Here's how the part is built. I have some questions about the finished solid (model axes, mm). Face numbers are marked on the shaded views. A direction names the side the tool comes from. Give positions to 0.01 mm unless a question says otherwise; leave off trailing zeros. Loops run counter-clockwise (first coordinate to the right, second up) from the corner with the lowest first, then second, coordinate; pieces in that order, holes last. Notation, with made-up numbers: (41.5, 85.25) - (84.5, 85.25) arc R24 cw to (84.5, 105.25) - close; hole circle Ø2 at (12, 60). An arc over 180 degrees is marked (long way). Use one line per item in the form item = value.
from build123d import *

# Parameters (mm, degrees)
SKETCH1_W                     = 63.5
SKETCH1_H                     = 63.5
BOSS_EXTRUDE1_DEPTH           = 50.8
SKETCH2_R                     = 2.54
BOSS_EXTRUDE2_DEPTH           = 12.7
SKETCH3_R                     = 12.7
BOSS_EXTRUDE3_DEPTH           = 15.24
BOSS_EXTRUDE3_TAPER           = 9
BOSS_EXTRUDE3_OTHER_WAY_DEPTH = 10.16
BOSS_EXTRUDE3_OTHER_WAY_TAPER = -9
BOSS_EXTRUDE4_START           = -25.4
SKETCH4_R                     = 18.536300075
BOSS_EXTRUDE4_DEPTH           = 3.175
BOSS_EXTRUDE4_TAPER           = 58
CHAMFER1_SIZE                 = 1.27
CHAMFER1_SIZE_2               = 1.527812426
SKETCH6_W                     = 38.1
SKETCH6_H                     = 10.16
BOSS_EXTRUDE6_DEPTH           = 6.35
BOSS_EXTRUDE7_DEPTH           = 6.35
BOSS_EXTRUDE7_DEPTH_BACK      = 6.35
SKETCH7_W                     = 1.5875
SKETCH7_H                     = 12.7
FILLET1_R                     = 1.27
SKETCH8_R                     = 4.445
CUT_EXTRUDE1_DEPTH            = 7.62


with BuildPart() as part:
    # Sketch1 → Boss-Extrude1 (new body)
    with BuildSketch(Plane.XY):
        Rectangle(SKETCH1_W, SKETCH1_H)
    extrude(amount=BOSS_EXTRUDE1_DEPTH)

    # Sketch2 → Boss-Extrude2 (add)
    with BuildSketch(Plane(origin=(0, 0, 0), x_dir=(-1, 0, 0), z_dir=(0, 0, -1))):
        with Locations(Location((0, 0, 0), (0, 0, 180))):
            Circle(SKETCH2_R)
    extrude(amount=BOSS_EXTRUDE2_DEPTH)

    # Sketch3 → Boss-Extrude3 (add)
    with BuildSketch(Plane(origin=(0, 0, -12.7), x_dir=(-1, 0, 0), z_dir=(0, 0, -1))):
        Circle(SKETCH3_R)
    extrude(amount=BOSS_EXTRUDE3_DEPTH, taper=BOSS_EXTRUDE3_TAPER)

    # Sketch3 → Boss-Extrude3 other way (add)
    with BuildSketch(Plane(origin=(0, 0, -12.7), x_dir=(-1, 0, 0), z_dir=(0, 0, -1))):
        Circle(SKETCH3_R)
    extrude(amount=-BOSS_EXTRUDE3_OTHER_WAY_DEPTH, taper=BOSS_EXTRUDE3_OTHER_WAY_TAPER)

    # Sketch4 → Boss-Extrude4 (add)
    with BuildSketch(Plane(origin=(0, 0, -27.94), x_dir=(-1, 0, 0), z_dir=(0, 0, -1)).offset(BOSS_EXTRUDE4_START)):
        Circle(SKETCH4_R)
    extrude(amount=BOSS_EXTRUDE4_DEPTH, taper=BOSS_EXTRUDE4_TAPER)

    # Chamfer1
    # the kernel refuses this chamfer: 1.527812426, 1.27 mm, written as the material it takes off along each edge
    with BuildSketch(Plane(origin=(0, 0, -27.94), x_dir=(-1, 0, 0), z_dir=(0, 1, 0))) as chamfer1_piece_1:
        Polygon((10.286221129 + CHAMFER1_SIZE * 0.15643446504, CHAMFER1_SIZE * 0.987688340595), (10.286221129 - CHAMFER1_SIZE_2, 0), (10.286221129, 0), align=None)
    revolve(axis=Axis((0, 0, -27.94), (0, 0, 1)), mode=Mode.SUBTRACT)

    # Sketch6 → Boss-Extrude6 (add)
    with BuildSketch(Plane.XY.offset(50.8)):
        with Locations((0, 14.933737581)):
            Rectangle(SKETCH6_W, SKETCH6_H)
    extrude(amount=BOSS_EXTRUDE6_DEPTH)

    # Sketch7 → Boss-Extrude7 (add, two sides: drawn at the far end of the back side and taken through both)
    with BuildSketch(Plane.XY.offset(57.15).offset(-BOSS_EXTRUDE7_DEPTH_BACK)):
        with Locations((-9.557292348, 14.933737581)):
            Rectangle(SKETCH7_W, SKETCH7_H)
        with Locations((-0.131236763, 14.933737581)):
            Rectangle(SKETCH7_W, SKETCH7_H)
        with Locations((10.440040529, 14.933737581)):
            Rectangle(SKETCH7_W, SKETCH7_H)
    extrude(amount=BOSS_EXTRUDE7_DEPTH + BOSS_EXTRUDE7_DEPTH_BACK)

    # Fillet1
    fillet1_edges = [part.edges().sort_by_distance(p)[0] for p in [
        (10.440040529, 21.283737581, 63.5),
        (10.440040529, 8.583737581, 63.5),
        (-0.131236763, 21.283737581, 63.5),
        (-0.131236763, 8.583737581, 63.5),
        (-9.557292348, 21.283737581, 63.5),
        (-9.557292348, 8.583737581, 63.5),
    ]]
    fillet(fillet1_edges, radius=FILLET1_R)

    # Sketch8 → Cut-Extrude1 (cut)
    with BuildSketch(Plane(origin=(0, 31.75, 0), x_dir=(1, 0, 0), z_dir=(0, 1, 0))):
        with Locations(Location((9.570348057, -25.239963614, 0), (0, 0, 270))):
            Circle(SKETCH8_R)
    extrude(amount=-CUT_EXTRUDE1_DEPTH, mode=Mode.SUBTRACT)


solid = part.part
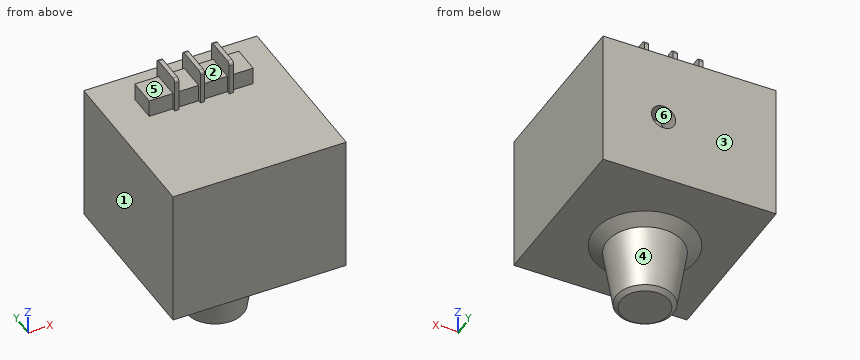
(1) If we section it at D-D (z = -15): List the corners of the cut face in (x, y) for me, plus the area to 3 significant figures.
Geometry says:
outline = circle Ø24.67 at (0, 0)
area = 478 mm²
(2) For P1, Ø0.8, axis at x = 10.5, z = 55.5, coming from the -Y side; P2, Ø12, axis at x = -9.5, y = -22.5, coming from the -Z side; P3, Ø0.8, axis at x = -9.5, z = 55, coming from the +Y side, each with a flat end and sliding along its axis, tell me the tip position at first contact or that it passes through.
Geometry says:
P1 = 8.58
P2 = -2.61
P3 = 21.28
(3) Thinking about a two-plate mould opening in X: for the marked faces 1, 2 and 3, which applies, pulls with the +X half, pulls with the -X half, needs draft (parallel to the pull), parting line crosses it, or undercut?
Geometry says:
face_1 = pulls with the -X half
face_2 = undercut
face_3 = needs draft
(4) If we section it at B-B (x = -23.5): List the corners of the cut face in (y, z) for me.
Geometry says:
outline = (-31.75, 0) - (31.75, 0) - (31.75, 50.8) - (-31.75, 50.8) - close
(5) If we section it at A-A (y = 26): List the corners of the cut face in (x, z) for me (3 decimals).
Geometry says:
outline = (-31.75, 0) - (31.75, 0) - (31.75, 50.8) - (-31.75, 50.8) - close; hole circle Ø8.89 at (9.57, 25.24)
(6) If I drill on probe 1 along Z at (x, y) = (-6, 2.5); probe 2 along Z at (x, y) = (-23, -10.5); probe 3 along Y at (x, z) = (13, 53), over which ranges is the centre line in solid material (lowest first)?
Geometry says:
probe_1 = -27.94 to -2.54, 0 to 50.8
probe_2 = 0 to 50.8
probe_3 = 9.85 to 20.01
(7) For the marked faces 4, 5 and 6, which set-ups out of +Z, -Z, +X, -X, +Y, -Y let a thin tool reach every point of the face, with its end or its side?
Geometry says:
face_4 = -Z
face_5 = +Z, -X, +Y, -Y
face_6 = +Y
